```python
from build123d import *

# Parameters (mm, degrees)
F0_W     = 42
F0_H     = 42
F0_R     = 1.5
F0_R_2   = 11
F0_R_3   = 2.5
F1_DEPTH = 40
F2_DEPTH = 2
F3_DEPTH = 24
F4_SIZE  = 5


with BuildPart() as f1:
    # F0 (on Front) → F1 (new body)
    with BuildSketch(Plane.XZ):
        Rectangle(F0_W, F0_H)
        with Locations((-15.5, -15.5)):
            Circle(F0_R, mode=Mode.SUBTRACT)
        with Locations((15.5, -15.5)):
            Circle(F0_R, mode=Mode.SUBTRACT)
        with Locations((-15.5, 15.5)):
            Circle(F0_R, mode=Mode.SUBTRACT)
        Circle(F0_R_2, mode=Mode.SUBTRACT)
        with Locations((15.5, 15.5)):
            Circle(F0_R, mode=Mode.SUBTRACT)
        Circle(F0_R_2)
        Circle(F0_R_3, mode=Mode.SUBTRACT)
        Circle(F0_R_3)
    extrude(amount=-F1_DEPTH)

    # F0 (on Front) → F2 (join)
    with BuildSketch(Plane.XZ):
        Circle(F0_R_2)
        Circle(F0_R_3, mode=Mode.SUBTRACT)
    extrude(amount=F2_DEPTH)

    # F0 (on Front) → F3 (join)
    with BuildSketch(Plane.XZ):
        Circle(F0_R_3)
    extrude(amount=F3_DEPTH)

    # F4
    f4_edges = [f1.edges().sort_by_distance(p)[0] for p in [
        (-21, 20, -21),
        (-21, 20, 21),
        (21, 20, 21),
        (21, 20, -21),
    ]]
    chamfer(f4_edges, length=F4_SIZE)


solid = f1.part
```
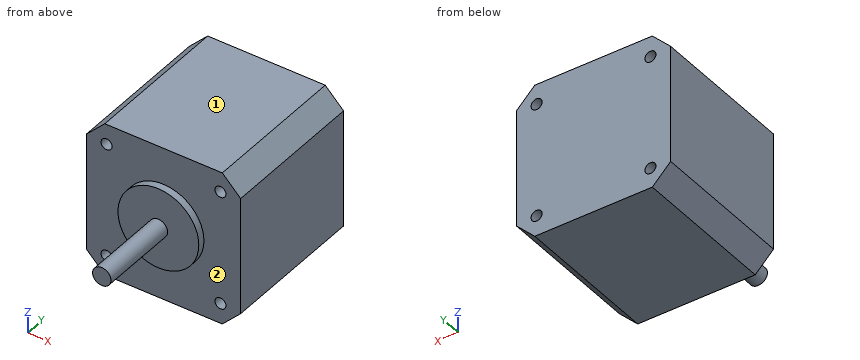
Geometry check sheet. Reference: the model listing, model coordinates, mm. Face numbers are marked on the shaded views. A direction names the side the tool comes from. Coordinates: 2 decimals unless noted, no trailing zeros. Loops run counter-clockwise (first coordinate to the right, second up) from the corner with the lowest first, then second, coordinate; pieces in that order, holes last.
Item 1: Thickness scan on line 1 (Z direction, x = 15.5, y = 14.5); line 2 (X direction, y = 25, z = 15). Record the ranges inside material, lowest first.
Item 2: Sectioned sample at C-C, the plane x = -15. Record the boundary of the cut face in (y, z), then the cut area to 3 significant figures.
Item 3: Go/stop test with flat-tipped pins: pin 1 Ø17.5 at (x, z) = (-4, -5) entering from -Y; pin 2 Ø4 at (x, z) = (-16, 7) entering from -Y; pin 3 Ø3 at (x, z) = (-5, -4.5) entering from -Y. Record where each tip stops, or that it passes through.
Item 4: Access from +Z, -Z, +X, -X, +Y, -Y to the whole of each face (thin tool, end or side, straight path). Record for the marked faces 1 and 2.
Item 5: Sectioned sample at B-B, the plane z = 0. Record the boundary of the cut face in (x, y).
Item 6: Sectioned sample at D-D, the plane x = 18. Record the boundary of the cut face in (y, z).
Item 7: Sectioned sample at A-A, the plane y = 24.5. Record the boundary of the cut face in (x, z), then the cut area to 3 significant figures.
Check result:
1. line 1: z = -21 to -17, -14 to 14, 17 to 21
1. line 2: x = -21 to -16.91, -14.09 to 14.09, 16.91 to 21
2. outline: (0, -21) - (40, -21) - (40, -16.91) - (0, -16.91) - close; (0, -14.09) - (40, -14.09) - (40, 14.09) - (0, 14.09) - close; (0, 16.91) - (40, 16.91) - (40, 21) - (0, 21) - close
2. area: 1,450 mm2
3. pin 1: stops at y = -24
3. pin 2: stops at y = 0
3. pin 3: stops at y = -2
4. face 1: +Z, +X, -X, +Y, -Y
4. face 2: -Y
5. outline: (-21, 0) - (-11, 0) - (-11, -2) - (-2.5, -2) - (-2.5, -24) - (2.5, -24) - (2.5, -2) - (11, -2) - (11, 0) - (21, 0) - (21, 40) - (-21, 40) - close
6. outline: (0, -19) - (40, -19) - (40, 19) - (0, 19) - close
7. outline: (-21, -16) - (-16, -21) - (16, -21) - (21, -16) - (21, 16) - (16, 21) - (-16, 21) - (-21, 16) - close; hole circle Ø3 at (-15.5, -15.5); hole circle Ø3 at (-15.5, 15.5); hole circle Ø3 at (15.5, -15.5); hole circle Ø3 at (15.5, 15.5)
7. area: 1,690 mm2
